The listing builds one solid part. Answer for the finished solid, in the listing's coordinates (mm). Give positions to 0.01 mm unless a question says otherwise; leave off trailing zeros. Order: outer loops, then holes, each group sorted by start corner. A loop starts at its lowest first (then second) coordinate and runs counter-clockwise, first axis right, second up. Notation, with made-up numbers: (45.5, 26.25) -> (79.5, 26.25) arc R17 ccw to (79.5, 58.25) -> close; hole circle Ø4 at (-4, 55.5). An arc over 180 degrees is marked (long way). One line per question, with ' | ' between items. Start each with the question number.
```python
from build123d import *

# Parameters (mm, degrees)
FR4_DEPTH                           = 1.7526
SKETCH7_R                           = 1.905
CUT_EXTRUDE1_DEPTH                  = 143.1375095
SKETCH8_R                           = 0.55
SKETCH8_R_2                         = 0.35
CONTROLLED_DEPTH_HOLES_TOP_DEPTH    = 1.1176
SKETCH9_R                           = 0.55
SKETCH9_R_2                         = 0.35
CONTROLLED_DEPTH_HOLES_BOTTOM_DEPTH = 1.1176


with BuildPart() as part:
    # Sketch1 → FR4 (new body)
    with BuildSketch(Plane(origin=(0, 0, 0), x_dir=(1, 0, 0), z_dir=(0, 1, 0))):
        with BuildLine():
            Line((0, 0), (110, 0))
            Line((110, 0), (110, 87))
            Line((110, 87), (104, 87))
            ThreePointArc((104, 87), (102.585786438, 87.585786438), (102, 89))
            Line((102, 89), (102, 90))
            Line((102, 90), (64, 90))
            Line((64, 90), (64, 89))
            ThreePointArc((64, 89), (63.414213562, 87.585786438), (62, 87))
            Line((62, 87), (48, 87))
            ThreePointArc((48, 87), (46.585786438, 87.585786438), (46, 89))
            Line((46, 89), (46, 90))
            Line((46, 90), (8, 90))
            Line((8, 90), (8, 89))
            ThreePointArc((8, 89), (7.414213562, 87.585786438), (6, 87))
            Line((6, 87), (0, 87))
            Line((0, 87), (0, 0))
        make_face()
    extrude(amount=FR4_DEPTH)

    # Sketch7 → Cut-Extrude1 (cut, through all)
    with BuildSketch(Plane(origin=(0, 1.7526, 0), x_dir=(1, 0, 0), z_dir=(0, 1, 0))):
        with Locations(Location((3.5, 15, 0), (0, 0, 270))):
            Circle(SKETCH7_R)
        with Locations(Location((106.5, 15, 0), (0, 0, 270))):
            Circle(SKETCH7_R)
        with Locations(Location((106.5, 30, 0), (0, 0, 270))):
            Circle(SKETCH7_R)
        with Locations(Location((106.5, 45, 0), (0, 0, 270))):
            Circle(SKETCH7_R)
        with Locations(Location((106.5, 60, 0), (0, 0, 270))):
            Circle(SKETCH7_R)
        with Locations(Location((106.5, 75, 0), (0, 0, 270))):
            Circle(SKETCH7_R)
        with Locations(Location((3.5, 30, 0), (0, 0, 270))):
            Circle(SKETCH7_R)
        with Locations(Location((3.5, 45, 0), (0, 0, 270))):
            Circle(SKETCH7_R)
        with Locations(Location((3.5, 60, 0), (0, 0, 270))):
            Circle(SKETCH7_R)
        with Locations(Location((3.5, 75, 0), (0, 0, 270))):
            Circle(SKETCH7_R)
    extrude(amount=-CUT_EXTRUDE1_DEPTH, mode=Mode.SUBTRACT)

    # Sketch8 → controlled-depth-holes.top (cut)
    with BuildSketch(Plane(origin=(0, 1.7526, 0), x_dir=(1, 0, 0), z_dir=(0, 1, 0))):
        with Locations(Location((8.9, 9.8, 0), (0, 0, 270))):
            Circle(SKETCH8_R)
        with Locations(Location((60.9, 9.8, 0), (0, 0, 270))):
            Circle(SKETCH8_R)
        with Locations(Location((60.9, 54.3, 0), (0, 0, 270))):
            Circle(SKETCH8_R)
        with Locations(Location((8.9, 54.3, 0), (0, 0, 270))):
            Circle(SKETCH8_R)
        with Locations(Location((49.1, 9.8, 0), (0, 0, 270))):
            Circle(SKETCH8_R_2)
        with Locations(Location((101.1, 9.8, 0), (0, 0, 270))):
            Circle(SKETCH8_R_2)
        with Locations(Location((101.1, 54.3, 0), (0, 0, 270))):
            Circle(SKETCH8_R_2)
        with Locations(Location((49.1, 54.3, 0), (0, 0, 270))):
            Circle(SKETCH8_R_2)
    extrude(amount=-CONTROLLED_DEPTH_HOLES_TOP_DEPTH, mode=Mode.SUBTRACT)

    # Sketch9 → controlled-depth-holes.bottom (cut)
    with BuildSketch(Plane.XZ):
        with Locations(Location((8.9, -9.5, 0), (0, 0, 270))):
            Circle(SKETCH9_R)
        with Locations(Location((60.9, -9.5, 0), (0, 0, 270))):
            Circle(SKETCH9_R)
        with Locations(Location((60.9, -54, 0), (0, 0, 270))):
            Circle(SKETCH9_R)
        with Locations(Location((8.9, -54, 0), (0, 0, 270))):
            Circle(SKETCH9_R)
        with Locations(Location((49.1, -9.5, 0), (0, 0, 270))):
            Circle(SKETCH9_R_2)
        with Locations(Location((101.1, -9.5, 0), (0, 0, 270))):
            Circle(SKETCH9_R_2)
        with Locations(Location((101.1, -54, 0), (0, 0, 270))):
            Circle(SKETCH9_R_2)
        with Locations(Location((49.1, -54, 0), (0, 0, 270))):
            Circle(SKETCH9_R_2)
    extrude(amount=-CONTROLLED_DEPTH_HOLES_BOTTOM_DEPTH, mode=Mode.SUBTRACT)


solid = part.part
```
(1) The part is cut by section A-A on x = 106.5. Determine the outline of the cut face in (y, z) (3 decimals).
(2) Consider line 1 (X direction, y = 0.85, z = -45) (3 decimals); line 2 (Z direction, x = 8.9, y = 0.55); line 3 (Z direction, x = 60.9, y = 0.95). Determine where each line is inside the solid, lowest interval first.
(3) Determine the mould class of faces 1 (the face through (54, 1.753, -46)), 2 (the face through (4.072, 0.889, -13.183)) for opening direction X: pulls with the +X half, pulls with the -X half, needs draft (parallel to the pull), parting line crosses it, or undercut.
(4) The part is cut by section B-B on y = 1.4. State how many separate pieces and enclosed holes the cut face has, plus the area to 3 significant figures.
(5) Given P1, Ø0.5, axis at y = 1, z = -89.5, coming from the +X side; P2, Ø0.9, axis at x = 55.5, y = 0.5, coming from the -Z side, each flat-ended and moving along its own axis, determine where each tip first touches the part or whether it passes through.
Result sheet:
1) outline: (0, -87) -> (1.753, -87) -> (1.753, -76.905) -> (0, -76.905) -> close; (0, -73.095) -> (1.753, -73.095) -> (1.753, -61.905) -> (0, -61.905) -> close; (0, -58.095) -> (1.753, -58.095) -> (1.753, -46.905) -> (0, -46.905) -> close; (0, -43.095) -> (1.753, -43.095) -> (1.753, -31.905) -> (0, -31.905) -> close; (0, -28.095) -> (1.753, -28.095) -> (1.753, -16.905) -> (0, -16.905) -> close; (0, -13.095) -> (1.753, -13.095) -> (1.753, 0) -> (0, 0) -> close
2) line 1: x = 0 to 1.595, 5.405 to 104.595, 108.405 to 110 | line 2: z = -90 to -54.55, -53.45 to -10.05, -8.95 to 0 | line 3: z = -87 to -54.85, -53.45 to -10.35, -8.95 to 0
3) face 1: needs draft | face 2: undercut
4) separate pieces: 1 | enclosed holes: 18 | area: 9,680 mm^2
5) P1: stops at x = 102 | P2: stops at z = -87
